Input: part model. Units: mm. Frame: model coordinates. A direction names the side the tool comes from. Coordinates: 2 decimals unless noted, no trailing zeros. Order: outer loops, then holes, each group sorted by start corner. A loop starts at its lowest first (then second) coordinate and runs counter-clockwise, first axis right, second up. Notation, with made-up numbers: (82.5, -0.5) -> (104.5, -0.5) arc R27 ccw to (104.5, 17.5) -> close; hole circle Ø1 at (-7.75, 40). An arc over 180 degrees is marked (long way). One line per question, with ' | ' between items.
```python
from build123d import *

# Parameters (mm, degrees)
F1_DEPTH = 10


with BuildPart() as f1:
    # F0 (on Top) → F1 (new body)
    with BuildSketch(Plane.XY):
        with BuildLine():
            ThreePointArc((-47.023135, 19.481115), (-46.730242, 20.188222), (-46.023135, 20.481115))
            Line((-46.023135, 20.481115), (-42.023135, 20.481115))
            ThreePointArc((-42.023135, 20.481115), (-41.316028, 20.188222), (-41.023135, 19.481115))
            Line((-41.023135, 19.481115), (-41.023135, 11.481115))
            ThreePointArc((-41.023135, 11.481115), (-40.730242, 10.774009), (-40.023135, 10.481115))
            Line((-40.023135, 10.481115), (-39.023135, 10.481115))
            ThreePointArc((-39.023135, 10.481115), (-38.316028, 10.774009), (-38.023135, 11.481115))
            Line((-38.023135, 11.481115), (-38.023135, 23.481115))
            ThreePointArc((-38.023135, 23.481115), (-38.316028, 24.188222), (-39.023135, 24.481115))
            Line((-39.023135, 24.481115), (-49.023135, 24.481115))
            ThreePointArc((-49.023135, 24.481115), (-49.730242, 24.188222), (-50.023135, 23.481115))
            Line((-50.023135, 23.481115), (-50.023135, 11.481115))
            ThreePointArc((-50.023135, 11.481115), (-49.730242, 10.774009), (-49.023135, 10.481115))
            Line((-49.023135, 10.481115), (-48.023135, 10.481115))
            ThreePointArc((-48.023135, 10.481115), (-47.316028, 10.774009), (-47.023135, 11.481115))
            Line((-47.023135, 11.481115), (-47.023135, 19.481115))
        make_face()
    extrude(amount=F1_DEPTH)


solid = f1.part
```
1. Ray query, line 1 (X direction, y = 18, z = 2.5); line 2 (Y direction, x = -43, z = 9.25); line 3 (X direction, y = 19.75, z = 6.5). Return the intervals inside material, ascending. Write a range as [from, to].
Recorded:
line 1: x = [-50.02, -47.02], [-41.02, -38.02] | line 2: y = [20.48, 24.48] | line 3: x = [-50.02, -46.99], [-41.06, -38.02]
2. Cut plane C-C, the plane x = -42.75. Return loops of the section in (y, z).
Recorded:
outline: (20.48, 0) -> (24.48, 0) -> (24.48, 10) -> (20.48, 10) -> close
3. Mould query, pull axis X, two halves, no side actions, for faces 1 (the face through (-49.738, 10.782, 4.93)), 2 (the face through (-47.023, 15, 5)), 3 (the face through (-44, 24.481, 5)). Classes: released by +X, released by -X, zero draft, split by the parting line, or undercut.
Recorded:
face 1: released by -X | face 2: undercut | face 3: zero draft
4. Cut plane D-D, the plane x = -47.25. Return loops of the section in (y, z), and give its area (3 significant figures).
Recorded:
outline: (10.85, 0) -> (24.48, 0) -> (24.48, 10) -> (10.85, 10) -> close | area: 136 mm^2
5. Cut plane B-B, the plane z = 0.5. Return loops of the section in (x, y).
Recorded:
outline: (-50.02, 11.48) arc R1 ccw to (-49.02, 10.48) -> (-48.02, 10.48) arc R1 ccw to (-47.02, 11.48) -> (-47.02, 19.48) arc R1 cw to (-46.02, 20.48) -> (-42.02, 20.48) arc R1 cw to (-41.02, 19.48) -> (-41.02, 11.48) arc R1 ccw to (-40.02, 10.48) -> (-39.02, 10.48) arc R1 ccw to (-38.02, 11.48) -> (-38.02, 23.48) arc R1 ccw to (-39.02, 24.48) -> (-49.02, 24.48) arc R1 ccw to (-50.02, 23.48) -> close
6. Pin query (flat end, axial travel): pin 1 Ø2 at (x, z) = (-44, 3) entering from -Y. Return the tip coordinate at first contact, or that it passes through.
Recorded:
pin 1: stops at y = 20.48
7. Access query for faces 4 (the face through (-49.72, 24.2, 4.93)), 5 (the face through (-46.74, 20.18, 4.93)). Directions: +Z, -Z, +X, -X, +Y, -Y. A direction counts if a zero-diameter tool reaches every point of the face in a straight line with its end or side. Return the directions, or none.
Recorded:
face 4: +Z, -Z, -X, +Y | face 5: +Z, -Z, -Y
8. Cut plane A-A, the plane y = 14.5. Return loops of the section in (x, z), and give its area (3 significant figures).
Recorded:
outline: (-50.02, 0) -> (-47.02, 0) -> (-47.02, 10) -> (-50.02, 10) -> close; (-41.02, 0) -> (-38.02, 0) -> (-38.02, 10) -> (-41.02, 10) -> close | area: 60.0 mm^2
